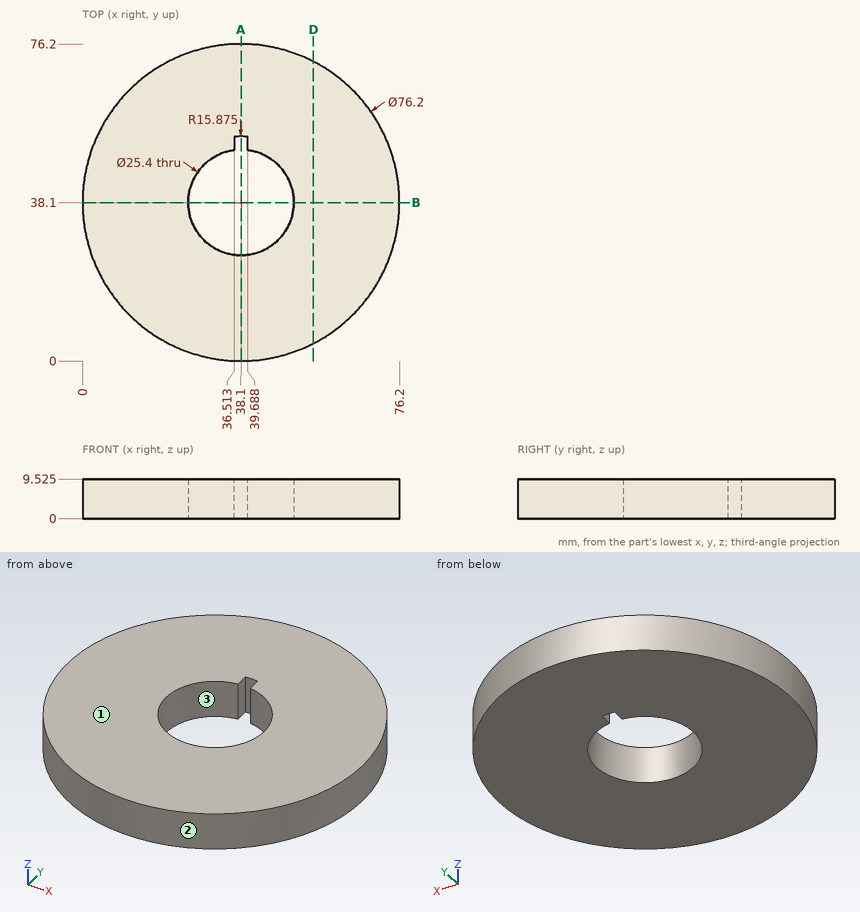
Input: dimensioned drawing with shaded views. Units: mm. Origin: part minimum x, y, z. Coordinates: 2 decimals unless noted, no trailing zeros. Order: outer loops, then holes, each group sorted by start corner. A loop starts at its lowest first (then second) coordinate and runs counter-clockwise, first axis right, second up. Notation, with made-up numbers: M -33.75,-29 L 15.25,-29 A16 cw 15.25,-18 Z; hole C 38,-21 d3. An arc over 180 degrees is marked long. Write each question's results on one line, items separated by ' | '. Start each with the question number.
Item 1: First-contact query: pin 1 Ø1.5 at (y, z) = (29.5, 4.5) entering from +X; pin 2 Ø2.5 at (y, z) = (52.5, 2.5) entering from -X; pin 3 Ø1 at (y, z) = (51.5, 4) entering from +X. Flat tips, straight axial feed; report the tip coordinate or a pass-through.
Item 2: Line query: probe 1 along Y at (x, z) = (38.1, 6.5) (1 decimal); probe 2 along Y at (x, z) = (65.5, 2) (1 decimal); probe 3 along X at (y, z) = (29, 3.5) (1 decimal). Output: solid intervals per line, ascending.
Item 3: Cut plane A-A (x = 38.1). Return loops of the section in (y, z) (1 decimal).
Item 4: Cut plane D-D (x = 55.5). Return loops of the section in (y, z) (1 decimal), and give its area (3 significant figures).
Item 5: Cut plane B-B (y = 38.1). Return loops of the section in (x, z) (1 decimal).
Item 6: Draft query along X for the marked faces 1, 2 and 3. Return one class per face: pulls with the +X half, pulls with the -X half, needs draft (parallel to the pull), parting line crosses it, or undercut.
Checked values:
1) pin 1: stops at x = 75.38 | pin 2: stops at x = 2.34 | pin 3: stops at x = 73.95
2) probe 1: y = 0 to 25.4, 54 to 76.2 | probe 2: y = 11.6 to 64.6 | probe 3: x = 1.1 to 29.2, 47 to 75.1
3) outline: M 0,0 L 25.4,0 L 25.4,9.5 L 0,9.5 Z; M 54,0 L 76.2,0 L 76.2,9.5 L 54,9.5 Z
4) outline: M 4.2,0 L 72,0 L 72,9.5 L 4.2,9.5 Z | area: 646 mm2
5) outline: M 0,0 L 25.4,0 L 25.4,9.5 L 0,9.5 Z; M 50.8,0 L 76.2,0 L 76.2,9.5 L 50.8,9.5 Z
6) face 1: needs draft | face 2: parting line crosses it | face 3: undercut
